Can you work these out from the model? Positions are in its coordinate system, mm. A direction names the side the tool comes from. Give positions to 0.01 mm unless a question says otherwise; leave off trailing zeros. Write each loop counter-clockwise with the first axis right and the second up, starting at its lowest first coordinate (ties: lowest second). Pieces come first, ordered by that corner, then holes.
1. On a 3-axis mill with a long thin cutter (end or side, diameter ignored), from which of +Z, -Z, +X, -X, +Y, -Y can I reach the whole of each face in a straight line? I mean faces 5 (the cylindrical face through (20.253, 0.132, -0.479)), 6 (the flat face through (0, -1.2, -3)). Say none if no direction works.
2. Suppose I cut it at A-A (z = -1). Please give me the cut outline in (x, y), and give its area (3 significant figures).
3. Suppose I cut it at D-D (y = 10). Please give me the cut outline in (x, z), and give its area (3 significant figures).
4. If I drill on probe 1 along Y at (x, z) = (-1, -1); probe 2 along Y at (x, z) = (14, -0.5); probe 3 along Y at (x, z) = (23.5, -3), over which ranges is the centre line in solid material (lowest first)?
5. I'm going to push flat-ended pins straight in: pin 1 (2.5 mm diameter, centred on y = 4.5, z = -2.5, fed in from +X); pin 2 (1.8 mm diameter, centred on x = 22.5, y = -1, fed in from +Z); pin 3 (1.8 mm diameter, centred on x = 2.5, z = -3, fed in from -Y). Where does each tip first touch, or does it pass through?
6. Suppose I cut it at C-C (x = -8). Please give me the cut outline in (y, z), and give its area (3 significant figures).
7. Suppose I cut it at B-B (x = -23.25). Please give me the cut outline in (y, z) (3 decimals).
8. Thinking about a two-plate mould opening in X: for faces 1 (the cylindrical face through (-30.55, -23.43, -2.96)), 2 (the flat face through (-18.4, -4, -3)), 3 (the flat face through (0, -6, -3)), 4 (the flat face through (-1, 1, -6)), which applies, pulls with the +X half, pulls with the -X half, needs draft (parallel to the pull), parting line crosses it, or undercut?
```python
from build123d import *

# Parameters (mm, degrees)
SKETCH1_R                  = 38.5
SKETCH1_R_2                = 1.925
SKETCH1_W                  = 36.8
SKETCH1_H                  = 4.8
MAIN_FLANGE_COUPLING_DEPTH = 6
SKETCH2_R                  = 38.5
SKETCH2_R_2                = 1.7
SKETCH2_W                  = 38.9
SKETCH2_H                  = 41.9
BOSS_EXTRUDE1_DEPTH        = 1
SKETCH3_R                  = 3
CUT_EXTRUDE1_DEPTH         = 3


with BuildPart() as part:
    # Sketch1 → Main Flange Coupling (new body)
    with BuildSketch(Plane.XY):
        Circle(SKETCH1_R)
        with Locations((-23.25, 0)):
            Circle(SKETCH1_R_2, mode=Mode.SUBTRACT)
        with Locations((23.25, 0)):
            Circle(SKETCH1_R_2, mode=Mode.SUBTRACT)
        with Locations((0, 4.4)):
            Rectangle(SKETCH1_W, SKETCH1_H, mode=Mode.SUBTRACT)
        with Locations((0, -3.6)):
            Rectangle(SKETCH1_W, SKETCH1_H, mode=Mode.SUBTRACT)
    extrude(amount=-MAIN_FLANGE_COUPLING_DEPTH)

    # Sketch2 → Boss-Extrude1 (add)
    with BuildSketch(Plane.XY):
        with Locations((0.65, -0.25)):
            Circle(SKETCH2_R)
        with Locations((-23.25, 0)):
            Circle(SKETCH2_R_2, mode=Mode.SUBTRACT)
        with Locations((23.25, 0)):
            Circle(SKETCH2_R_2, mode=Mode.SUBTRACT)
        with Locations((0.2, -0.2)):
            Rectangle(SKETCH2_W, SKETCH2_H, mode=Mode.SUBTRACT)
    extrude(amount=BOSS_EXTRUDE1_DEPTH)

    # Sketch3 → Cut-Extrude1 (cut)
    with BuildSketch(Plane.XY.offset(1)):
        with Locations((-23.25, 0)):
            Circle(SKETCH3_R)
        with Locations((23.25, 0)):
            Circle(SKETCH3_R)
    extrude(amount=-CUT_EXTRUDE1_DEPTH, mode=Mode.SUBTRACT)


solid = part.part
```
Checks:
1. face 5: +Z
1. face 6: +Z, -Z
2. outline: circle Ø77 at (0, 0); hole circle Ø6 at (-23.25, 0); hole (-18.4, -6) - (18.4, -6) - (18.4, -1.2) - (-18.4, -1.2) - close; hole (-18.4, 2) - (18.4, 2) - (18.4, 6.8) - (-18.4, 6.8) - close; hole circle Ø6 at (23.25, 0)
2. area: 4,250 mm2
3. outline: (-37.18, -6) - (37.18, -6) - (37.18, 0) - (37.76, 0) - (37.76, 1) - (19.65, 1) - (19.65, 0) - (-19.25, 0) - (-19.25, 1) - (-36.46, 1) - (-36.46, 0) - (-37.18, 0) - close
3. area: 481 mm2
4. probe 1: y = -38.49 to -6, -1.2 to 2, 6.8 to 38.49
4. probe 2: y = -35.86 to -6, -1.2 to 2, 6.8 to 35.86
4. probe 3: y = -30.5 to -1.91, 1.91 to 30.5
5. pin 1: stops at x = 38.36
5. pin 2: stops at z = -2
5. pin 3: stops at y = -38.47
6. outline: (-37.77, 0) - (-37.66, 0) - (-37.66, -6) - (-6, -6) - (-6, 0) - (-21.15, 0) - (-21.15, 1) - (-37.77, 1) - close; (-1.2, -6) - (2, -6) - (2, 0) - (-1.2, 0) - close; (6.8, -6) - (37.66, -6) - (37.66, 0) - (37.27, 0) - (37.27, 1) - (20.75, 1) - (20.75, 0) - (6.8, 0) - close
6. area: 427 mm2
7. outline: (-30.687, -6) - (-1.925, -6) - (-1.925, -2) - (-3, -2) - (-3, 1) - (-30.433, 1) - (-30.433, 0) - (-30.687, 0) - close; (1.925, -6) - (30.687, -6) - (30.687, 0) - (29.933, 0) - (29.933, 1) - (3, 1) - (3, -2) - (1.925, -2) - close
8. face 1: parting line crosses it
8. face 2: undercut
8. face 3: undercut
8. face 4: needs draft
